Model file for the job. Use its own axes, mm. Give positions to 0.01 mm unless a question says otherwise; leave off trailing zeros. Loops run counter-clockwise (first coordinate to the right, second up) from the corner with the lowest first, then second, coordinate; pieces in that order, holes last. Notation, with made-up numbers: (21, 73) -> (80, 73) arc R22 cw to (80, 108) -> close; hole circle Ø6 at (-1.5, 60.25). An arc over 180 degrees is marked (long way). Use CSV: the item, a comma, the result in double quotes. Start each with the question number.
(1) Flat gauge pins, fed straight in: pin 1 (1.5 mm diameter, centred on x = 6, y = 1.5, fed in from +Z); pin 2 (1.5 mm diameter, centred on x = 4, y = 2, fed in from -Z); pin 3 (1.5 mm diameter, centred on y = 1.5, z = -39, fed in from +X). Where does each tip first touch, or does it go through?
(2) Cut at C-C on x = 8.5. Write the cut outline in (y, z).
(3) Cut at B-B on y = 0.85. State how many separate pieces and enclosed holes the cut face has, then the cut area to 3 significant figures.
(4) Drill centre lines: probe 1 along Z at (x, y) = (25, 1.1); probe 2 along Z at (x, y) = (70, 1.8); probe 3 along X at (y, z) = (0.95, -5.5). Where is each one in solid material? Low to high.
(5) Cut at A-A on x = 36. Write the cut outline in (y, z), then the cut area to 3 significant figures.
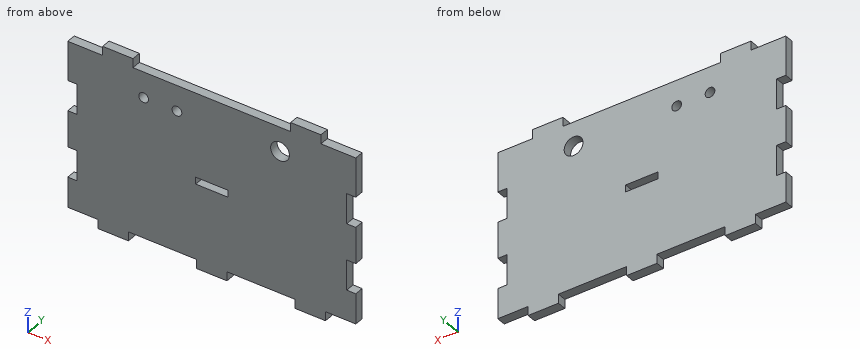
Autodesk Inventor part; units mm, degrees
ref_plane "YZ Plane" through (0, 0, 0) normal (1, 0, 0) x (0, 1, 0)
ref_plane "XZ Plane" through (0, 0, 0) normal (0, 1, 0) x (-1, 0, 0)
ref_plane "XY Plane" through (0, 0, 0) normal (0, 0, 1) x (1, 0, 0)
sketch "Parede_lateral_1" plane through (0, 0, 0) normal (0, 1, 0) x (-1, 0, 0)
  line L0 (0, 0) -> (-95, 0)
  line L1 (-95, 0) -> (-95, -52)
  line L2 (-95, -52) -> (0, -52)
  line L3 (0, -52) -> (0, 0)
  circle A0 centre (-70, -5) radius 3.1
  dimension "d0" = 95
  dimension "d1" = 52
  dimension "d101" = 6.2
  dimension "d102" = 5
  dimension "d105" = 25
extrude "Extrusão1" add sketch "Parede_lateral_1" along normal blind 3 contours L3 L2 L1 L0 | A0
sketch "Esboço3" plane through (0, 3, 0) normal (0, 1, 0) x (1, 0, 0)
  line L0 (42.1875, 27.15) -> (52.8125, 27.15)
  line L1 (52.8125, 27.15) -> (52.8125, 24.85)
  line L2 (52.8125, 24.85) -> (42.1875, 24.85)
  line L3 (42.1875, 24.85) -> (42.1875, 27.15)
  line L4 (95, 52) -> (0, 52)
  line L5 (95, 0) -> (95, 52)
  point P0 (0, 0)
  point P1 (46, 52)
  point P2 (27, 52)
  point P3 (47.5, 27.15)
  point P4 (95, 26)
  point P5 (52.8125, 26)
  dimension "d26" = 10.625
  dimension "d27" = 2.3
  dimension "d30" = 24.85
  dimension "d31" = 42.1875
extrude "Extrusão3" cut sketch "Esboço3" against normal blind 10
sketch "Esboço4" plane through (0, 3, 0) normal (0, 1, 0) x (1, 0, 0)
  line L0 (95, 52) -> (0, 52)
  line L1 (0, 52) -> (0, 0)
  line L2 (10, 52) -> (20, 52)
  line L3 (20, 52) -> (20, 55)
  line L4 (20, 55) -> (10, 55)
  line L5 (10, 55) -> (10, 52)
  line L6 (42.5, 52) -> (52.5, 52)
  line L7 (52.5, 52) -> (52.5, 55)
  line L8 (52.5, 55) -> (42.5, 55)
  line L9 (42.5, 55) -> (42.5, 52)
  line L10 (75, 52) -> (85, 52)
  line L11 (85, 52) -> (85, 55)
  line L12 (85, 55) -> (75, 55)
  line L13 (75, 55) -> (75, 52)
  line L14 (0, 0) -> (95, 0)
  line L15 (95, 0) -> (95, 52)
  dimension "d43" = 3
  dimension "d74" = 3
  dimension "d75" = 3
extrude "Extrusão4" add sketch "Esboço4" against normal blind 3 contours L0 L13 L12 L11 | L0 L9 L8 L7 | L5 L4 L3 L0
sketch "Esboço5" plane through (0, 3, 0) normal (0, 1, 0) x (1, 0, 0)
  line L0 (0, 10) -> (3, 10)
  line L1 (3, 10) -> (3, 20)
  line L2 (3, 20) -> (0, 20)
  line L3 (0, 20) -> (0, 10)
  line L4 (0, 32) -> (3, 32)
  line L5 (3, 32) -> (3, 42)
  line L6 (3, 42) -> (0, 42)
  line L7 (0, 42) -> (0, 32)
  line L8 (10, 52) -> (0, 52)
  line L9 (0, 0) -> (95, 0)
  line L10 (95, 0) -> (95, 52)
  line L11 (95, 10) -> (92, 10)
  line L12 (92, 10) -> (92, 20)
  line L13 (92, 20) -> (95, 20)
  line L14 (95, 20) -> (95, 10)
  line L15 (95, 42) -> (92, 42)
  line L16 (92, 42) -> (92, 32)
  line L17 (92, 32) -> (95, 32)
  line L18 (95, 32) -> (95, 42)
  line L19 (95, 52) -> (85, 52)
  line L20 (0, 0) -> (95, 0)
  point P0 (1.5, 42)
  point P1 (10, 0)
  point P2 (93.5, 42)
  point P3 (85, 0)
  point P4 (93.5, 10)
  point P5 (92, 37)
  point P6 (95, 37)
  dimension "d63" = 3
  dimension "d64" = 10
  dimension "d65" = 3
  dimension "d66" = 10
  dimension "d67" = 10
  dimension "d68" = 10
  dimension "d71" = 10
  dimension "d72" = 10
  dimension "d76" = 3
  dimension "d77" = 3
extrude "Extrusão5" cut sketch "Esboço5" against normal blind 3
sketch "Esboço6" plane through (0, 0, 0) normal (0, -1, 0) x (1, 0, 0)
  line L0 (0, 0) -> (95, 0)
  line L1 (95, 0) -> (95, 3)
  line L2 (95, 3) -> (0, 3)
  line L3 (0, 3) -> (0, 0)
  dimension "d79" = 95
  dimension "d80" = 3
extrude "Extrusão6" add sketch "Esboço6" against normal blind 3
sketch "Esboço7" plane through (0, 0, 0) normal (0, -1, 0) x (1, 0, 0)
  line L0 (95, 3) -> (0, 3)
  line L1 (11.5, 3) -> (21.5, 3)
  line L2 (21.5, 3) -> (21.5, 6)
  line L3 (21.5, 6) -> (11.5, 6)
  line L4 (11.5, 6) -> (11.5, 3)
  line L5 (83.5, 3) -> (73.5, 3)
  line L6 (73.5, 3) -> (73.5, 6)
  line L7 (73.5, 6) -> (83.5, 6)
  line L8 (83.5, 6) -> (83.5, 3)
  line L9 (0, -10) -> (0, 3)
  line L10 (95, 3) -> (95, -10)
  point P0 (0, 0)
  point P1 (11.5, 4.5)
  point P2 (95, -3.5)
  point P3 (83.5, 4.5)
  point P4 (21.5, 3)
  dimension "d83" = 10
  dimension "d84" = 3
  dimension "d85" = 10
  dimension "d86" = 3
  dimension "d87" = 11.5
  dimension "d88" = 11.5
extrude "Extrusão7" add sketch "Esboço7" against normal blind 3
sketch "Esboço8" plane through (0, 3, 0) normal (0, 1, 0) x (1, 0, 0)
  circle A0 centre (25, 5.5) radius 1.6
  circle A1 centre (36, 5.5) radius 1.6
  line L0 (21.5, -3) -> (73.5, -3)
  line L1 (0, 10) -> (0, -3)
  point P0 (0, 0)
  dimension "d92" = 3.2
  dimension "d93" = 3.2
  dimension "d94" = 11
  dimension "d95" = 8.5
  dimension "d96" = 8.5
  dimension "d98" = 25
extrude "Extrusão8" cut sketch "Esboço8" against normal blind 10
extrude "Extrusão9" cut sketch "Parede_lateral_1" along normal blind 10 contours A0
properties part number "Parede_lateral_1"
Check result:
1,pin 1,"z = 3"
1,pin 2,"z = -52"
1,pin 3,"x = 92"
2,outline,"(0, -52) -> (3, -52) -> (3, 3) -> (0, 3) -> close"
3,separate pieces,"1"
3,enclosed holes,"4"
3,area,"5,180 mm²"
4,probe 1,"-52 to -7.1, -3.9 to 3"
4,probe 2,"-52 to -8.1, -1.9 to 3"
4,probe 3,"0 to 23.4, 26.6 to 34.4, 37.6 to 66.94, 73.06 to 95"
5,outline,"(0, -52) -> (3, -52) -> (3, -7.1) -> (0, -7.1) -> close; (0, -3.9) -> (3, -3.9) -> (3, 3) -> (0, 3) -> close"
5,area,"155 mm²"
